Check sheet for the modelled part. Datum: model origin and axes. Units: mm. Face numbers are marked on the shaded views. A direction names the side the tool comes from. Give positions to 0.01 mm unless a question says otherwise; leave off trailing zeros. Loops run counter-clockwise (first coordinate to the right, second up) from the corner with the lowest first, then second, coordinate; pieces in that order, holes last. Notation, with made-up numbers: M 52,52 L 78,52 A23 cw 78,64 Z; hole C -39.75,21 d2. An arc over 180 degrees is marked long. Write each question's results on one line, items separated by ' | '. Start each with the question number.
1. Sectioned sample at D-D on x = 10. Record the cut outline in (y, z).
2. Go/stop test with flat-tipped pins: pin 1 (5 mm diameter, centred on x = 4.5, y = 8, fed in from -Z); pin 2 (1.4 mm diameter, centred on x = 1, z = 18.95, fed in from -Y); pin 3 (3 mm diameter, centred on y = 11, z = 11.5, fed in from +X); pin 4 (1 mm diameter, centred on x = 12.5, y = -0.5, fed in from +Z). Record where each tip stops, or that it passes through.
3. Sectioned sample at B-B on x = 20. Give the number of separate pieces and of enclosed holes in the cut face, and give its area (3 significant figures).
4. Sectioned sample at A-A on y = 0. Record the cut outline in (x, z), and give its area (3 significant figures).
5. Tool access check on the marked faces 1, 2, 3 and 4. Record the directions out of +Z, -Z, +X, -X, +Y, -Y that give a thin tool (end or side, any length) a straight path to the whole face; none if there is none.
6. Draft check along X on the marked faces 5, 6 and 7. Enter one of: pulls with the +X half, pulls with the -X half, needs draft (parallel to the pull), parting line crosses it, or undercut.
7. Sectioned sample at C-C on z = 15. Record the cut outline in (x, y).
8. Material ranges on line 1 along X through (y, z) = (20, 7.95); line 2 along Y through (x, z) = (0, 7.45); line 3 along Y through (x, z) = (10, 18), recorded low to high.
```python
from build123d import *

# Parameters (mm, degrees)
SKETCH1_W                  = 30
SKETCH1_H                  = 30
SKETCH1_R                  = 1.6
SKETCH1_W_2                = 70
SKETCH1_H_2                = 12
BOSS_EXTRUDE1_DEPTH        = 6
SKETCH1_3_W                = 30
SKETCH1_3_H                = 30
SKETCH1_3_R                = 1.6
BOSS_EXTRUDE2_DEPTH        = 22.33
CUT_EXTRUDE1_DEPTH         = 78.612040947
SKETCH3_R                  = 2.55
CUT_EXTRUDE2_DEPTH         = 8
CUT_EXTRUDE3_DEPTH         = 4.5
SKETCH6_R                  = 5
CUT_EXTRUDE5_DEPTH         = 8.6
SKETCH7_R                  = 1.6
CUT_EXTRUDE6_DEPTH         = 101.740403513
SKETCH8_R                  = 2.85
CUT_EXTRUDE7_DEPTH         = 11
BOSS_EXTRUDE3_START        = 2.43
SKETCH9_R                  = 3.4
SKETCH9_R_2                = 2.55
BOSS_EXTRUDE3_DEPTH        = 2.43
CHAMFER1_SIZE              = 1.2
FILLET3_R                  = 4
CHAMFER2_SIZE              = 0.8
CUT_EXTRUDE8_DEPTH         = 3
CHAMFER3_SIZE              = 0.8
LPATTERN1_COUNT            = 3
LPATTERN1_PITCH            = 25
CHAMFER3_OF_LPATTERN1_SIZE = 0.8
SKETCH12_W                 = 103.210606925
SKETCH12_H                 = 33.832940417
CUT_EXTRUDE9_DEPTH         = 6
SKETCH13_R                 = 0.8
CUT_EXTRUDE10_DEPTH        = 5


with BuildPart() as part:
    # Sketch1 → Boss-Extrude1 (new body)
    # profile 1 of 2: a face of its own
    with BuildSketch(Plane.XY):
        with Locations((10, 10)):
            Rectangle(SKETCH1_W, SKETCH1_H)
        with Locations((20, 0)):
            Circle(SKETCH1_R, mode=Mode.SUBTRACT)
        with Locations((20, 20)):
            Circle(SKETCH1_R, mode=Mode.SUBTRACT)
        with Locations((0, 20)):
            Circle(SKETCH1_R, mode=Mode.SUBTRACT)
        Circle(SKETCH1_R, mode=Mode.SUBTRACT)
    # profile 2 of 2: a face of its own
    with BuildSketch(Plane.XY):
        with Locations((60, 10)):
            Rectangle(SKETCH1_W_2, SKETCH1_H_2)
    extrude(amount=BOSS_EXTRUDE1_DEPTH)

    # Sketch1<3> → Boss-Extrude2 (add)
    with BuildSketch(Plane.XY):
        with Locations((10, 10)):
            Rectangle(SKETCH1_3_W, SKETCH1_3_H)
        with Locations((20, 0)):
            Circle(SKETCH1_3_R, mode=Mode.SUBTRACT)
        with Locations((20, 20)):
            Circle(SKETCH1_3_R, mode=Mode.SUBTRACT)
        with Locations((0, 20)):
            Circle(SKETCH1_3_R, mode=Mode.SUBTRACT)
        Circle(SKETCH1_3_R, mode=Mode.SUBTRACT)
    extrude(amount=BOSS_EXTRUDE2_DEPTH)

    # Sketch2 → Cut-Extrude1 (cut, through all)
    with BuildSketch(Plane(origin=(25, 0, 0), x_dir=(0, 0, -1), z_dir=(1, 0, 0))):
        with BuildLine():
            Line((-6.515476918, 16.231667643), (-9.112158418, 16.231667643))
            Line((-9.112158418, 16.231667643), (-10.20449761, 16.039058771))
            ThreePointArc((-10.20449761, 16.039058771), (-11.275650893, 14.693383456), (-12.742453793, 15.59154862))
            Line((-12.742453793, 15.59154862), (-13.786185118, 15.407510627))
            Line((-13.786185118, 15.407510627), (-13.786185118, 4.591753459))
            Line((-13.786185118, 4.591753459), (-12.742453793, 4.407715465))
            ThreePointArc((-12.742453793, 4.407715465), (-11.275650893, 5.305880629), (-10.20449761, 3.960205314))
            Line((-10.20449761, 3.960205314), (-9.112158418, 3.767596443))
            Line((-9.112158418, 3.767596443), (-6.515476918, 3.767596443))
            Line((-6.515476918, 3.767596443), (-5.902540869, 3.767596443))
            Line((-5.902540869, 3.767596443), (-5.902540869, 16.231667643))
            Line((-5.902540869, 16.231667643), (-6.515476918, 16.231667643))
        make_face()
    extrude(amount=-CUT_EXTRUDE1_DEPTH, mode=Mode.SUBTRACT)

    # Sketch3 → Cut-Extrude2 (cut)
    with BuildSketch(Plane.XY.offset(22.33)):
        with Locations((10, 10)):
            Circle(SKETCH3_R)
    extrude(amount=-CUT_EXTRUDE2_DEPTH, mode=Mode.SUBTRACT)

    # Sketch5 → Cut-Extrude3 (cut)
    with BuildSketch(Plane(origin=(0, 0, 13.786185118), x_dir=(-1, 0, 0), z_dir=(0, 0, -1))):
        Polygon((-5.32346282, 10), (-7.66173141, 14.05), (-12.33826859, 14.05), (-14.67653718, 10), (-12.33826859, 5.95), (-7.66173141, 5.95), align=None)
    extrude(amount=-CUT_EXTRUDE3_DEPTH, mode=Mode.SUBTRACT)

    # Sketch6 → Cut-Extrude5 (cut)
    with BuildSketch(Plane(origin=(0, 0, 0), x_dir=(-1, 0, 0), z_dir=(0, 0, -1))):
        with Locations((-10, 10)):
            Circle(SKETCH6_R)
    extrude(amount=-CUT_EXTRUDE5_DEPTH, mode=Mode.SUBTRACT)

    # Sketch7 → Cut-Extrude6 (cut, through all)
    with BuildSketch(Plane(origin=(0, 0, 0), x_dir=(-1, 0, 0), z_dir=(0, 0, -1))):
        with BuildLine():
            ThreePointArc((-90.1, 10), (-88.5, 8.4), (-86.9, 10))
            Line((-86.9, 10), (-90.1, 10))
        make_face()
        with BuildLine():
            Line((-90.1, 10), (-86.9, 10))
            ThreePointArc((-86.9, 10), (-88.5, 11.6), (-90.1, 10))
        make_face()
        with Locations((-63.5, 10)):
            Circle(SKETCH7_R)
        with Locations((-38.5, 10)):
            Circle(SKETCH7_R)
    extrude(amount=-CUT_EXTRUDE6_DEPTH, mode=Mode.SUBTRACT)

    # Sketch8 → Cut-Extrude7 (cut)
    with BuildSketch(Plane.XY.offset(22.33)):
        with Locations((20, 20)):
            Circle(SKETCH8_R)
        with Locations((20, 0)):
            Circle(SKETCH8_R)
        Circle(SKETCH8_R)
        with Locations((0, 20)):
            Circle(SKETCH8_R)
    extrude(amount=-CUT_EXTRUDE7_DEPTH, mode=Mode.SUBTRACT)

    # Sketch9 → Boss-Extrude3 (add)
    with BuildSketch(Plane.XY.offset(22.33).offset(BOSS_EXTRUDE3_START)):
        with Locations(Location((10, 10, 0), (0, 0, 180))):
            Circle(SKETCH9_R)
        with Locations((10, 10)):
            Circle(SKETCH9_R_2, mode=Mode.SUBTRACT)
    extrude(amount=-BOSS_EXTRUDE3_DEPTH)

    # Chamfer1
    chamfer1_edges = [part.edges().sort_by_distance(p)[0] for p in [
        (13.4, 10, 22.33),
    ]]
    chamfer(chamfer1_edges, length=CHAMFER1_SIZE)

    # Fillet3
    # the kernel refuses this fillet: 4 mm, written as the material it adds along each edge
    with BuildSketch(Plane(origin=(25, 4, 0), x_dir=(0, -1, 0), z_dir=(0, 0, 1))) as fillet3_piece_1:
        with BuildLine():
            CenterArc((FILLET3_R, FILLET3_R), FILLET3_R, 180, 90)
            Line((0, FILLET3_R), (0, 0))
            Line((0, 0), (FILLET3_R, 0))
        make_face()
    extrude(amount=5.902540869)
    with BuildSketch(Plane(origin=(25, 16, 0), x_dir=(0, 1, 0), z_dir=(0, 0, 1))) as fillet3_piece_2:
        with BuildLine():
            CenterArc((FILLET3_R, -FILLET3_R), FILLET3_R, 90, 90)
            Line((0, -FILLET3_R), (0, 0))
            Line((0, 0), (FILLET3_R, 0))
        make_face()
    extrude(amount=5.902540869)
    # the kernel refuses this fillet: 4 mm, written as the material it takes off along each edge
    with BuildSketch(Plane(origin=(-5, -5, 32.33), x_dir=(1, 0, 0), z_dir=(0, 0, -1)), Plane(origin=(-5, 25, 32.33), x_dir=(0, -1, 0), z_dir=(0, 0, -1)), Plane(origin=(25, 25, -10), x_dir=(0, -1, 0), z_dir=(0, 0, 1)), Plane(origin=(25, -5, -10), x_dir=(-1, 0, 0), z_dir=(0, 0, 1))) as fillet3_2_piece_1:
        with BuildLine():
            CenterArc((FILLET3_R, -FILLET3_R), FILLET3_R, 90, 90)
            Line((0, -FILLET3_R), (0, 0))
            Line((0, 0), (FILLET3_R, 0))
        make_face()
    extrude(amount=42.33, mode=Mode.SUBTRACT)
    with BuildSketch(Plane(origin=(95, 16, -10), x_dir=(-1, 0, 0), z_dir=(0, 0, 1))) as fillet3_2_piece_2:
        with BuildLine():
            CenterArc((FILLET3_R, FILLET3_R), FILLET3_R, 180, 90)
            Line((0, FILLET3_R), (0, 0))
            Line((0, 0), (FILLET3_R, 0))
        make_face()
    extrude(amount=26, mode=Mode.SUBTRACT)
    with BuildSketch(Plane(origin=(95, 4, -10), x_dir=(-1, 0, 0), z_dir=(0, 0, 1))) as fillet3_2_piece_3:
        with BuildLine():
            CenterArc((FILLET3_R, -FILLET3_R), FILLET3_R, 90, 90)
            Line((0, -FILLET3_R), (0, 0))
            Line((0, 0), (FILLET3_R, 0))
        make_face()
    extrude(amount=26, mode=Mode.SUBTRACT)

    # Chamfer2
    chamfer2_edges = [part.edges().sort_by_distance(p)[0] for p in [
        (-2.85, 20, 22.33),
        (-2.85, 0, 22.33),
        (17.15, 0, 22.33),
        (17.15, 20, 22.33),
    ]]
    chamfer(chamfer2_edges, length=CHAMFER2_SIZE)

    # Sketch10 → Cut-Extrude8 (cut)
    with BuildSketch(Plane(origin=(0, 0, 0), x_dir=(-1, 0, 0), z_dir=(0, 0, -1))):
        Polygon((-85.266838493, 10), (-86.883419246, 12.8), (-90.116580754, 12.8), (-91.733161507, 10), (-90.116580754, 7.2), (-86.883419246, 7.2), align=None)
    cut_extrude8 = extrude(amount=-CUT_EXTRUDE8_DEPTH, mode=Mode.SUBTRACT)

    # Chamfer3
    chamfer3_edges = [part.edges().sort_by_distance(p)[0] for p in [
        (86.075128869, 8.6, 0),
        (86.075128869, 11.4, 0),
        (88.5, 12.8, 0),
        (90.924871131, 11.4, 0),
        (90.924871131, 8.6, 0),
        (88.5, 7.2, 0),
    ]]
    chamfer(chamfer3_edges, length=CHAMFER3_SIZE)

    # LPattern1: Cut-Extrude8 ×3
    with Locations(*[(-i * LPATTERN1_PITCH, 0, 0) for i in range(1, LPATTERN1_COUNT)]):
        add(cut_extrude8, mode=Mode.SUBTRACT)

    # Chamfer3 of LPattern1
    chamfer3_of_lpattern1_edges = [part.edges().sort_by_distance(p)[0] for p in [
        (61.075128869, 8.6, 0),
        (61.075128869, 11.4, 0),
        (63.5, 12.8, 0),
        (65.924871131, 11.4, 0),
        (65.924871131, 8.6, 0),
        (63.5, 7.2, 0),
        (36.075128869, 8.6, 0),
        (36.075128869, 11.4, 0),
        (38.5, 12.8, 0),
        (40.924871131, 11.4, 0),
        (40.924871131, 8.6, 0),
        (38.5, 7.2, 0),
    ]]
    chamfer(chamfer3_of_lpattern1_edges, length=CHAMFER3_OF_LPATTERN1_SIZE)

    # Sketch12 → Cut-Extrude9 (cut)
    with BuildSketch(Plane(origin=(0, 0, 0), x_dir=(-1, 0, 0), z_dir=(0, 0, -1))):
        with Locations((-45.050346637, 9.848960088)):
            Rectangle(SKETCH12_W, SKETCH12_H)
    extrude(amount=-CUT_EXTRUDE9_DEPTH, mode=Mode.SUBTRACT)

    # Sketch13 → Cut-Extrude10 (cut)
    with BuildSketch(Plane.XZ.offset(5)):
        with Locations(Location((1, 18.949828429, 0), (0, 0, 270))):
            Circle(SKETCH13_R)
        with Locations(Location((1, 12.449828429, 0), (0, 0, 270))):
            Circle(SKETCH13_R)
    extrude(amount=-CUT_EXTRUDE10_DEPTH, mode=Mode.SUBTRACT)


solid = part.part
```
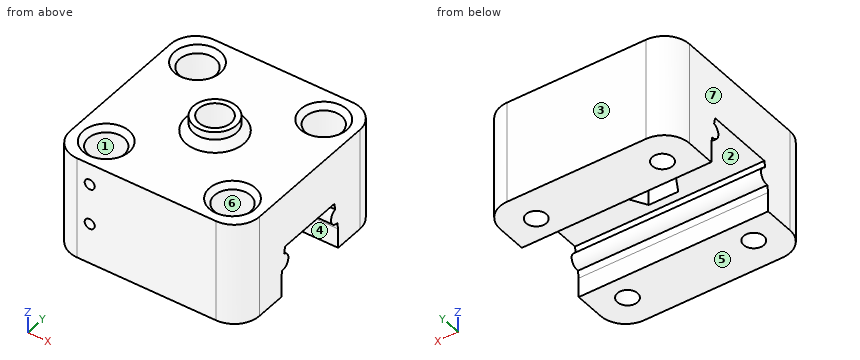
Output values:
1) outline: M -5,6 L 3.77,6 L 3.77,9.11 L 3.96,10.2 A1.3 ccw 4.41,12.74 L 4.59,13.79 L 5.95,13.79 L 5.95,18.29 L 7.45,18.29 L 7.45,24.76 L 6.6,24.76 L 6.6,23.53 L 5.4,22.33 L -5,22.33 Z; M 12.55,18.29 L 14.05,18.29 L 14.05,13.79 L 15.41,13.79 L 15.59,12.74 A1.3 ccw 16.04,10.2 L 16.23,9.11 L 16.23,6 L 25,6 L 25,22.33 L 14.6,22.33 L 13.4,23.53 L 13.4,24.76 L 12.55,24.76 Z
2) pin 1: z = 13.79 | pin 2: y = 2.29 | pin 3: through | pin 4: z = 22.33
3) separate pieces: 3 | enclosed holes: 0 | area: 240 mm2
4) outline: M -5,6 L -1.6,6 L -1.6,11.33 L -2.85,11.33 L -2.85,21.53 L -3.65,22.33 L -5,22.33 Z; M 1.6,6 L 18.4,6 L 18.4,11.33 L 17.15,11.33 L 17.15,21.53 L 16.35,22.33 L 3.65,22.33 L 2.85,21.53 L 2.85,11.33 L 1.6,11.33 Z; M 21.6,6 L 25,6 L 25,22.33 L 23.65,22.33 L 22.85,21.53 L 22.85,11.33 L 21.6,11.33 Z | area: 329 mm2
5) face 1: +Z | face 2: +X, -X | face 3: +Z, -Z, +X, -X, +Y | face 4: -Z, +X, -X
6) face 5: needs draft | face 6: undercut | face 7: pulls with the -X half
7) outline: M -5,-1 A4 ccw -1,-5 L 21,-5 A4 ccw 25,-1 L 25,21 A4 ccw 21,25 L -1,25 A4 ccw -5,21 Z; hole C 0,0 d5.7; hole C 0,20 d5.7; hole M 5.32,10 L 7.66,5.95 L 12.34,5.95 L 14.68,10 L 12.34,14.05 L 7.66,14.05 Z; hole C 20,0 d5.7; hole C 20,20 d5.7
8) line 1: -5 to -1.6, 1.6 to 18.4, 21.6 to 25 | line 2: -5 to -1.6, 1.6 to 3.77, 16.23 to 18.4, 21.6 to 25 | line 3: -5 to 5.95, 14.05 to 25
